```python
from build123d import *

# Parameters (mm, degrees)
SKETCH1_R           = 82.55
SKETCH1_R_2         = 74.93
SKETCH1_R_3         = 69.85
BOSS_EXTRUDE2_DEPTH = 6.35
SKETCH1_4_R         = 74.93
SKETCH1_4_R_2       = 69.85
BOSS_EXTRUDE3_DEPTH = 6.35
CUT_EXTRUDE1_DEPTH  = 3.175


with BuildPart() as part:
    # Sketch1 → Boss-Extrude2 (new body)
    # profile 1 of 3: a face of its own
    with BuildSketch(Plane(origin=(0, 0, 0), x_dir=(1, 0, 0), z_dir=(0, 1, 0))):
        with Locations(Location((0, 0, 0), (0, 0, 270))):
            Circle(SKETCH1_R)
        Circle(SKETCH1_R_2, mode=Mode.SUBTRACT)
    # profile 2 of 3: a face of its own
    with BuildSketch(Plane(origin=(0, 0, 0), x_dir=(1, 0, 0), z_dir=(0, 1, 0))):
        Circle(SKETCH1_R_2)
        Circle(SKETCH1_R_3, mode=Mode.SUBTRACT)
    # profile 3 of 3: a face of its own
    with BuildSketch(Plane(origin=(0, 0, 0), x_dir=(1, 0, 0), z_dir=(0, 1, 0))):
        Circle(SKETCH1_R_3)
    extrude(amount=BOSS_EXTRUDE2_DEPTH)

    # Sketch1_4 → Boss-Extrude3 (add)
    with BuildSketch(Plane(origin=(0, 0, 0), x_dir=(1, 0, 0), z_dir=(0, 1, 0))):
        with Locations(Location((0, 0, 0), (0, 0, 270))):
            Circle(SKETCH1_4_R)
        with Locations(Location((0, 0, 0), (0, 0, 270))):
            Circle(SKETCH1_4_R_2, mode=Mode.SUBTRACT)
    extrude(amount=-BOSS_EXTRUDE3_DEPTH)

    # Sketch2 → Cut-Extrude1 (cut)
    with BuildSketch(Plane(origin=(0, 6.35, 0), x_dir=(1, 0, 0), z_dir=(0, 1, 0))):
        with BuildLine():
            Line((-38.1, 19.05), (-38.1, -19.05))
            ThreePointArc((-38.1, -19.05), (-57.15, 0), (-38.1, 19.05))
        make_face()
        with BuildLine():
            Line((38.1, 19.05), (38.1, -19.05))
            ThreePointArc((38.1, -19.05), (57.15, 0), (38.1, 19.05))
        make_face()
    extrude(amount=-CUT_EXTRUDE1_DEPTH, mode=Mode.SUBTRACT)


solid = part.part
```
CAD build for the part. Positions are in the model's coordinates, mm. A direction names the side the tool comes from. Coordinates: 2 decimals unless noted, no trailing zeros. Order: outer loops, then holes, each group sorted by start corner. A loop starts at its lowest first (then second) coordinate and runs counter-clockwise, first axis right, second up. Notation, with made-up numbers: M 41,1.25 L 87,1.25 A32 ccw 87,38.25 Z; hole C 80,78.5 d11. An arc over 180 degrees is marked long. Answer as CSV lines item,"result".
1) Drill centre lines: L1, parallel to X at y = -4, z = 0; L2, parallel to Z at x = 10.5, y = -4.5; L3, parallel to Z at x = 1, y = 2. Where is each one in solid material? Low to high. Write a range as from..to.
Verdict:
L1,"-74.93..-69.85, 69.85..74.93"
L2,"-74.19..-69.06, 69.06..74.19"
L3,"-82.54..82.54"
2) Cut at B-B (x = -66). List the corners of the cut face in (y, z), then the cut area to 3 significant figures.
Verdict:
outline,"M -6.35,-35.48 L 0,-35.48 L 0,-49.58 L 6.35,-49.58 L 6.35,49.58 L 0,49.58 L 0,35.48 L -6.35,35.48 L -6.35,22.87 L 0,22.87 L 0,-22.87 L -6.35,-22.87 Z"
area,"790 mm2"
3) Cut at D-D (z = -43.5). List the corners of the cut face in (x, y).
Verdict:
outline,"M -70.16,0 L -61.01,0 L -61.01,-6.35 L -54.65,-6.35 L -54.65,0 L 54.65,0 L 54.65,-6.35 L 61.01,-6.35 L 61.01,0 L 70.16,0 L 70.16,6.35 L -70.16,6.35 Z"
4) Flat gauge pins, fed straight in: P1, Ø1.5, axis at y = -4, z = 8, coming from the +X side; P2, Ø8, axis at x = 50.5, z = -8, coming from the +Y side (3 decimals); P3, Ø1.6, axis at y = 4, z = -3, coming from the +X side. Where does each tip first touch, or does it go through?
Verdict:
P1,"x = 74.58"
P2,"y = 3.175"
P3,"x = 82.52"
5) Cut at C-C (y = -2.5). List the corners of the cut face in (x, z), then the cut area to 3 significant figures.
Verdict:
outline,"C 0,0 d149.86; hole C 0,0 d139.7"
area,"2,310 mm2"
6) Cut at A-A (z = 0). List the corners of the cut face in (x, y) (3 decimals).
Verdict:
outline,"M -82.55,0 L -74.93,0 L -74.93,-6.35 L -69.85,-6.35 L -69.85,0 L 69.85,0 L 69.85,-6.35 L 74.93,-6.35 L 74.93,0 L 82.55,0 L 82.55,6.35 L 57.15,6.35 L 57.15,3.175 L 38.1,3.175 L 38.1,6.35 L -38.1,6.35 L -38.1,3.175 L -57.15,3.175 L -57.15,6.35 L -82.55,6.35 Z"
7) 3-axis set-ups, long thin cutter, end or side, ignore diameter. For faces 1 (the cylindrical face through (81.848, 3.131, -10.746)), 2 (the flat face through (-45, 3.175, 0)), 3 (the flat face through (-1, 0, -1)): which of +Z, -Z, +X, -X, +Y, -Y reach the whole face in a straight line?
Verdict:
face 1,"+Y, -Y"
face 2,"+Y"
face 3,"-Y"
8) Mould opens along Z. For faces 4 (the cylindrical face through (-68.2, -3.1, -15.1)), 5 (the cylindrical face through (-73.15, -3.13, -16.24)), 6 (the flat face through (45, 3.175, 0)), 7 (the flat face through (18, 0, 73)) say: released by +Z, released by -Z, zero draft, split by the parting line, or undercut.
Verdict:
face 4,"undercut"
face 5,"split by the parting line"
face 6,"undercut"
face 7,"zero draft"
